```python
from build123d import *

# Parameters (mm, degrees)
SKETCH1_R           = 22.499999958
SKETCH1_R_2         = 21.699999958
BOSS_EXTRUDE1_DEPTH = 92
SKETCH3_R           = 45.65
CUT_EXTRUDE1_DEPTH  = 8.6
SKETCH3_3_R         = 43.65
CUT_EXTRUDE2_DEPTH  = 7.6


with BuildPart() as part:
    # Sketch1 → Boss-Extrude1 (new body)
    with BuildSketch(Plane(origin=(0, 0, 0), x_dir=(0, 1, 0), z_dir=(0, 0, 1))):
        with Locations(Location((0, 0, 0), (0, 0, 270))):
            Circle(SKETCH1_R)
        with Locations(Location((0, 0, 0), (0, 0, 270))):
            Circle(SKETCH1_R_2, mode=Mode.SUBTRACT)
    extrude(amount=BOSS_EXTRUDE1_DEPTH)

    # Sketch3 → Cut-Extrude1 (cut)
    with BuildSketch(Plane.YZ):
        with Locations((0, 125)):
            Circle(SKETCH3_R)
    extrude(amount=-CUT_EXTRUDE1_DEPTH, mode=Mode.SUBTRACT)

    # Sketch3<3> → Cut-Extrude2 (cut)
    with BuildSketch(Plane.YZ):
        with Locations((0, 125)):
            Circle(SKETCH3_3_R)
    extrude(amount=CUT_EXTRUDE2_DEPTH, mode=Mode.SUBTRACT)


solid = part.part
```
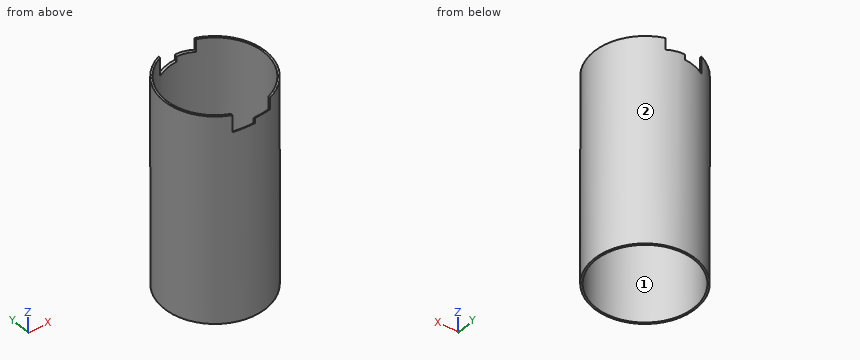
Source: CAD feature listing. Evaluate the final solid. Frame: model axes, mm. Face numbers are marked on the shaded views. Coordinates: 2 decimals unless noted, no trailing zeros. Write each loop counter-clockwise with the first axis right and the second up, starting at its lowest first coordinate (ties: lowest second). Pieces come first, ordered by that corner, then holes. Notation, with made-up numbers: (79, 25.25) -> (107, 25.25) arc R36 cw to (107, 60.25) -> close; hole circle Ø11 at (-16.5, 80.5). An arc over 180 degrees is marked (long way). Return JSON: item names as keys, results as strings. Group by question number.
1) Contact query for flat-ended pins moving along their axis: P1, Ø10, axis at x = -2, z = 10, coming from the -Y side; P2, Ø8, axis at y = -13, z = 39.5, coming from the -X side; P3, Ø1, axis at x = -3.5, z = 49.5, coming from the +Y side; P4, Ø8, axis at x = -13.5, y = -10.5, coming from the +Z side. Output: stop coordinate, or through.
2) Ray query, line 1 along Y through (x, z) = (0, 19); line 2 along Y through (x, z) = (-13, 65.5). Return the intervals inside material, ascending.
3) Section query C-C, the plane z = 46.5. Return loops of the section in (x, y), plus the area to 3 significant figures.
4) Section query B-B, the plane x = 2.5. Return loops of the section in (y, z), plus the area to 3 significant figures.
5) Mould query, pull axis Y, two halves, no side actions, for the marked faces 1 and 2. Classes: +Y half, -Y half, draft (parallel to the pull), parting line (faces both ways), or undercut.
6) Section query A-A, the plane y = 0. Return loops of the section in (x, z).
From the geometry:
{
 "1": {"P1": "y = -22.5", "P2": "x = -20.62", "P3": "y = 22.3", "P4": "through"},
 "2": {"line 1": "-22.5 to -21.7, 21.7 to 22.5", "line 2": "-18.36 to -17.37, 17.37 to 18.36"},
 "3": {"outline": "circle Ø45 at (0, 0); hole circle Ø43.4 at (0, 0)", "area": "111 mm²"},
 "4": {"outline": "(-22.36, 0) -> (-21.56, 0) -> (-21.56, 87.04) arc R43.65 cw to (-22.36, 87.51) -> close; (21.56, 0) -> (22.36, 0) -> (22.36, 87.51) arc R43.65 cw to (21.56, 87.04) -> close", "area": "141 mm²"},
 "5": {"face 1": "undercut", "face 2": "parting line"},
 "6": {"outline": "(-22.5, 0) -> (-21.7, 0) -> (-21.7, 92) -> (-22.5, 92) -> close; (21.7, 0) -> (22.5, 0) -> (22.5, 92) -> (21.7, 92) -> close"}
}
